Model file for the job. Use its own axes, mm. Coordinates: 2 decimals unless noted, no trailing zeros. Write each loop counter-clockwise with the first axis right and the second up, starting at its lowest first coordinate (ties: lowest second). Pieces come first, ordered by that corner, then holes.
Q1. Band-saw the part on A-A, the plane z = 154.5. Write the cut outline in (x, y), plus the area to 3 significant figures.
Q2. Drill centre lines: probe 1 along Y at (x, z) = (5.5, 26.5); probe 2 along Z at (x, y) = (1, 11.5) (3 decimals). Where is each one in solid material? Low to high.
Q3. Band-saw the part on C-C, the plane x = 6.5. Write the cut outline in (y, z).
Q4. Pin check, flat tips, straight feed: P1, Ø4, axis at x = 11, y = 3.5, coming from the -Z side; P2, Ø3, axis at y = 9, z = 100.5, coming from the +X side; P3, Ø4, axis at x = 5, z = 51.5, coming from the -Y side. Stop position of each tip, or through.
Q5. Band-saw the part on B-B, the plane y = 8.5. Write the cut outline in (x, z), plus the area to 3 significant figures.
from build123d import *

# Parameters (mm, degrees)
BOSS_EXTRUDE1_DEPTH     = 171.45
CUT_EXTRUDE1_DEPTH      = 173.299266975
CUT_EXTRUDE1_DEPTH_BACK = 173.299266975


with BuildPart() as part:
    # Sketch1 → Boss-Extrude1 (new body)
    with BuildSketch(Plane.XY):
        Polygon((0, 0), (0, 12.7), (1.27, 12.7), (1.27, 1.27), (12.7, 1.27), (12.7, 0), align=None)
    extrude(amount=BOSS_EXTRUDE1_DEPTH)

    # Sketch2 → Cut-Extrude1 (cut, two sides: drawn at the far end of the back side and taken through both)
    with BuildSketch(Plane(origin=(0, 1.27, 0), x_dir=(1, 0, 0), z_dir=(0, 1, 0)).offset(-CUT_EXTRUDE1_DEPTH_BACK)):
        Polygon((0, -168.047045256), (12.7, -171.45), (0, -171.45), align=None)
        Polygon((0, 0), (12.7, -12.7), (12.7, 0), align=None)
    extrude(amount=CUT_EXTRUDE1_DEPTH + CUT_EXTRUDE1_DEPTH_BACK, mode=Mode.SUBTRACT)


solid = part.part
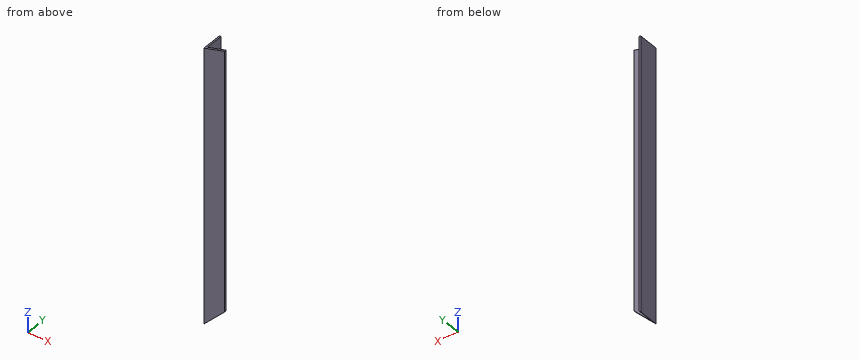
Answer sheet:
1. outline: (0, 0) - (12.7, 0) - (12.7, 1.27) - (1.27, 1.27) - (1.27, 12.7) - (0, 12.7) - close
1. area: 30.6 mm2
2. probe 1: y = 0 to 1.27
2. probe 2: z = 1 to 168.315
3. outline: (0, 6.5) - (1.27, 6.5) - (1.27, 169.79) - (0, 169.79) - close
4. P1: passes through
4. P2: stops at x = 1.27
4. P3: stops at y = 0
5. outline: (0, 0) - (1.27, 1.27) - (1.27, 168.39) - (0, 168.05) - close
5. area: 213 mm2
